Autodesk Inventor part; units mm, degrees
ref_plane "YZ Plane" through (0, 0, 0) normal (1, 0, 0) x (0, 1, 0)
ref_plane "XZ Plane" through (0, 0, 0) normal (0, 1, 0) x (-1, 0, 0)
ref_plane "XY Plane" through (0, 0, 0) normal (0, 0, 1) x (1, 0, 0)
sketch "Sketch1" plane through (0, 0, 0) normal (0, 0, 1) x (1, 0, 0)
  circle A0 centre (0, 0) radius 35
  circle A1 centre (0, 0) radius 18
  circle A2 centre (0, 0) radius 29 construction
  line L0 (0, 0) -> (0, 29) construction
  line L1 (0, 0) -> (20.5061, 20.5061) construction
  dimension "d0" = 70
  dimension "d1" = 36
  dimension "d2" = 58
  dimension "d3" = 45
extrude "Extrusion1" add sketch "Sketch1" along normal blind 5
hole "Hole1" at (20.5061, 20.5061, 0) direction (0, 0, 1) diameter 6.6 end through all
pattern_circular "Circular Pattern1" count 4 over 360 about axis through (0, 0, -10) along (0, 0, 1) of "Hole1"
chamfer "Chamfer1" distance 1 angle 45 2 edges at (-18, 0, 0) (-35, 0, 0)
properties part number "PWTR-0051"
Design review of the part built by this model. Coordinates are the model's own, in mm. Coordinates: 2 decimals unless noted, no trailing zeros. Loops run counter-clockwise (first coordinate to the right, second up) from the corner with the lowest first, then second, coordinate; pieces in that order, holes last. Notation, with made-up numbers: (69.25, 83.25) - (105.25, 83.25) arc R12 ccw to (105.25, 91.25) - close; hole circle Ø4 at (67.25, 56.5). An arc over 180 degrees is marked (long way). Use CSV: the item, a comma, the result in double quotes. Start each with the question number.
1) For pin 1 Ø2 at (y, z) = (-21.5, 2.5) entering from -X; pin 2 Ø1.5 at (x, z) = (-25, 4) entering from -Y; pin 3 Ø1.5 at (x, z) = (-19.5, 4) entering from +Y, all flat-tipped, find the tip position at first contact; note any pin that passes through.
2) The part is to be moulded in two halves that separate along Y. For faces 1 (the flat face through (15, -15, 0)), 2 (the cylindrical face through (-22.28, 17.724, 2.535)), 3 (the cylindrical face through (-28, 21, 3)), say which applies: +Y half, -Y half, draft (parallel to the pull), parting line (faces both ways), or undercut.
3) Consider section C-C on z = 3.45. Write out the cut boundary in (x, y).
4) Consider section A-A on x = 0. Write out the cut boundary in (y, z).
5) Wall thickness on L1, parallel to X at y = 22, z = 2.85; L2, parallel to X at y = 23.5, z = 2.45; L3, parallel to Y at x = 0, z = 3.95: over which ranges is each line inside the solid? List them lowest first. Write a range as from..to.
Geometry says:
1,pin 1,"x = -28.37"
1,pin 2,"y = -25.24"
1,pin 3,"y = 29.55"
2,face 1,"draft"
2,face 2,"undercut"
2,face 3,"parting line"
3,outline,"circle Ø70 at (0, 0); hole circle Ø6.6 at (-20.51, -20.51); hole circle Ø6.6 at (-20.51, 20.51); hole circle Ø36 at (0, 0); hole circle Ø6.6 at (20.51, -20.51); hole circle Ø6.6 at (20.51, 20.51)"
4,outline,"(-35, 1) - (-34, 0) - (-19, 0) - (-18, 1) - (-18, 5) - (-35, 5) - close; (18, 1) - (19, 0) - (34, 0) - (35, 1) - (35, 5) - (18, 5) - close"
5,L1,"-27.22..-23.45, -17.56..17.56, 23.45..27.22"
5,L2,"-25.94..-21.89, -19.12..19.12, 21.89..25.94"
5,L3,"-35..-18, 18..35"
